Source: three-view drawing plus pictorial views. Frame: mm from the lowest corner of the part. Coordinates: 2 decimals unless noted, no trailing zeros. Write each loop counter-clockwise with the first axis right and the second up, starting at its lowest first coordinate (ties: lowest second). Pieces come first, ordered by that corner, then holes. Notation, with made-up numbers: (3.5, 17) - (7.5, 17) arc R31 ccw to (7.5, 52) - close; hole circle Ø4 at (-6.5, 48.25). An arc over 180 degrees is marked (long way). Put each result on its own line as item: value. Start each with the question number.
1. Cut plane A-A, the plane x = 50.8. Return loops of the section in (y, z) (1 decimal), and give its area (3 significant figures).
2. Line query: line 1 (Z direction, x = 50.8, y = 1.55); line 2 (Z direction, x = 50.8, y = 2.3); line 3 (X direction, y = 1.5, z = 40.5). Output: solid intervals per line, ascending.
3. Cut plane C-C, the plane y = 2.6. Return loops of the section in (x, z).
4. Cut plane D-D, the plane x = 74. Return loops of the section in (y, z) (3 decimals), and give its area (3 significant figures).
5. Cut plane B-B, the plane z = 50.8. Return loops of the section in (x, y) (1 decimal), and give its area (3 significant figures).
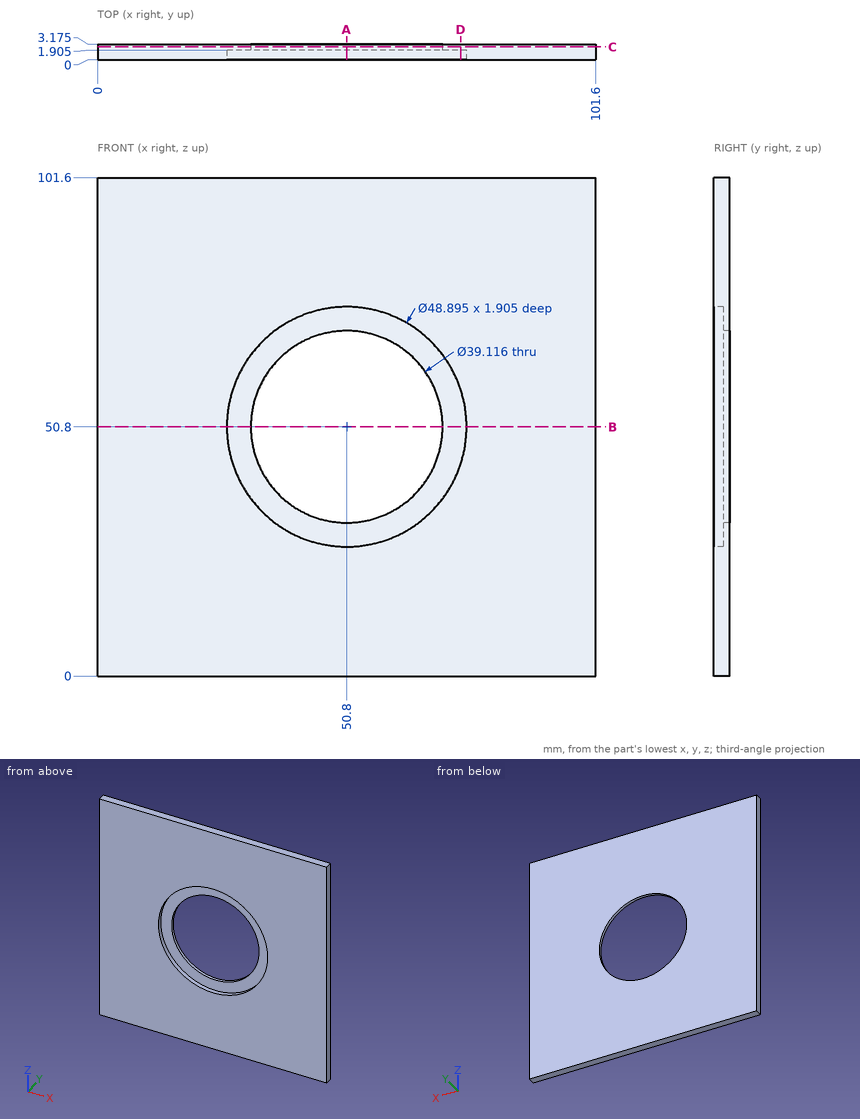
Report:
1. outline: (0, 0) - (3.2, 0) - (3.2, 31.2) - (1.9, 31.2) - (1.9, 26.4) - (0, 26.4) - close; (0, 75.2) - (1.9, 75.2) - (1.9, 70.4) - (3.2, 70.4) - (3.2, 101.6) - (0, 101.6) - close
1. area: 180 mm^2
2. line 1: z = 0 to 26.35, 75.25 to 101.6
2. line 2: z = 0 to 31.24, 70.36 to 101.6
2. line 3: x = 0 to 28.63, 72.97 to 101.6
3. outline: (0, 0) - (101.6, 0) - (101.6, 101.6) - (0, 101.6) - close; hole circle Ø39.12 at (50.8, 50.8)
4. outline: (0, 0) - (3.175, 0) - (3.175, 101.6) - (0, 101.6) - (0, 58.51) - (1.905, 58.51) - (1.905, 43.09) - (0, 43.09) - close
4. area: 293 mm^2
5. outline: (0, 0) - (26.4, 0) - (26.4, 1.9) - (31.2, 1.9) - (31.2, 3.2) - (0, 3.2) - close; (70.4, 1.9) - (75.2, 1.9) - (75.2, 0) - (101.6, 0) - (101.6, 3.2) - (70.4, 3.2) - close
5. area: 180 mm^2
